Verification items for this drawing (mm, ordinates from the low corner). A direction names the side the tool comes from. Coordinates: 2 decimals unless noted, no trailing zeros. Write each loop counter-clockwise with the first axis right and the second up, starting at its lowest first coordinate (ties: lowest second). Pieces come first, ordered by that corner, then holes. Notation, with made-up numbers: (-8, 55.5) -> (48, 55.5) arc R5 cw to (48, 64.5) -> close; hole circle Ø1 at (15, -23.5). An arc over 180 degrees is marked (long way). Use CSV: the item, a comma, the result in double quotes.
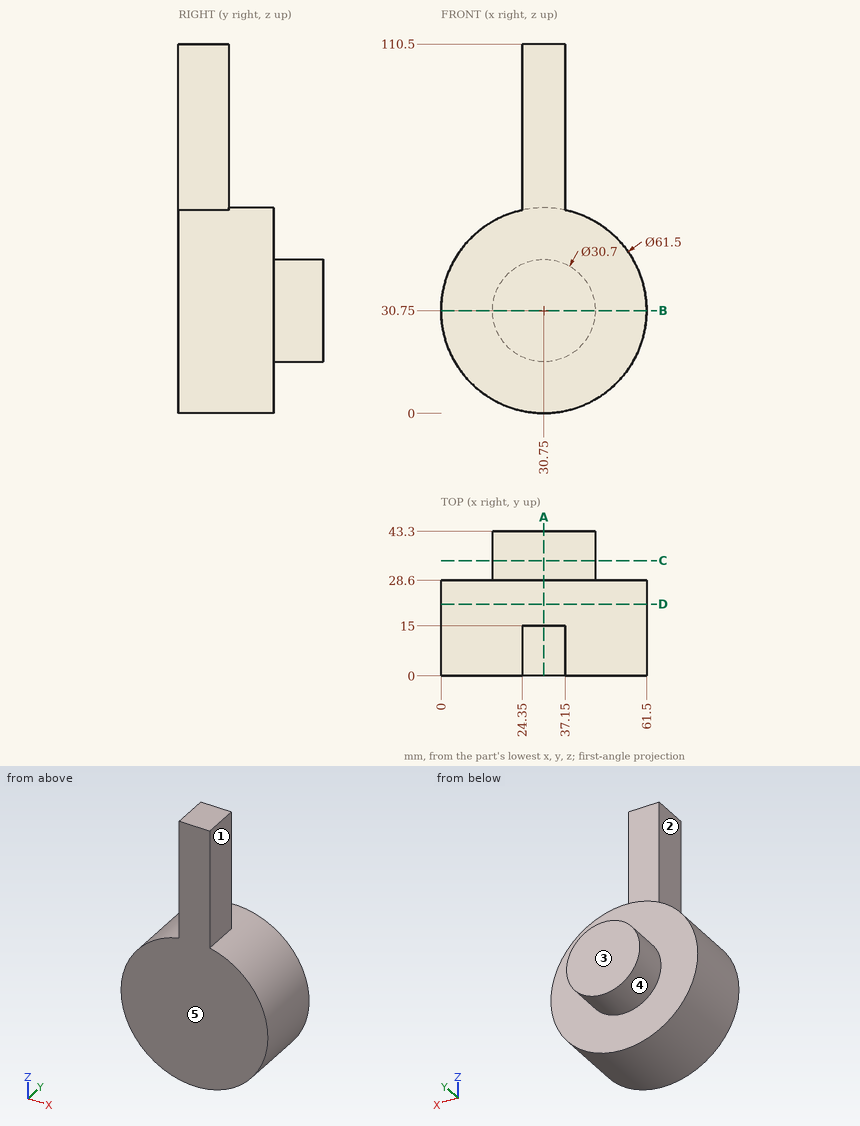
1) Cross-section at B-B (z = 30.75). Record the boundary of the cut face in (x, y), plus the area to 3 significant figures.
Return value:
outline,"(0, 0) -> (61.5, 0) -> (61.5, 28.6) -> (46.1, 28.6) -> (46.1, 43.3) -> (15.4, 43.3) -> (15.4, 28.6) -> (0, 28.6) -> close"
area,"2,210 mm2"
2) Cross-section at A-A (x = 30.75). Record the boundary of the cut face in (y, z), plus the area to 3 significant figures.
Return value:
outline,"(0, 0) -> (28.6, 0) -> (28.6, 15.4) -> (43.3, 15.4) -> (43.3, 46.1) -> (28.6, 46.1) -> (28.6, 61.5) -> (15, 61.5) -> (15, 110.5) -> (0, 110.5) -> close"
area,"2,950 mm2"
3) Gauge pin test, flat ends, axial feed: pin 1 (3 mm diameter, centred on x = 6.5, z = 34.5, fed in from +Y); pin 2 (10 mm diameter, centred on x = 29, z = 81, fed in from +Y); pin 3 (5 mm diameter, centred on y = 35, z = 32.5, fed in from -X). Record the tip position at first contact, or that the pin passes through.
Return value:
pin 1,"y = 28.6"
pin 2,"y = 15"
pin 3,"x = 15.4"
4) Scan lines: L1, parallel to X at y = 2, z = 90; L2, parallel to Z at x = 30, y = 23.5; L3, parallel to Y at x = 7, z = 49.5. Record each from-to range of solid material in increasing order.
Return value:
L1,"24.35 to 37.15"
L2,"0.01 to 61.49"
L3,"0 to 28.6"
5) Cross-section at D-D (y = 21.5). Record the boundary of the cut face in (x, z).
Return value:
outline,"circle Ø61.5 at (30.75, 30.75)"
6) Cross-section at C-C (y = 34.5). Record the boundary of the cut face in (x, z).
Return value:
outline,"circle Ø30.7 at (30.75, 30.75)"
7) Set-up check for the marked faces 1, 2, 3, 4 and 5: record each of +Z, -Z, +X, -X, +Y, -Y from which the full face is reachable in a straight line by a thin tool's end or side.
Return value:
face 1,"+Z, +X, +Y, -Y"
face 2,"+Z, -X, +Y, -Y"
face 3,"+Z, -Z, +X, -X, +Y"
face 4,"+Y"
face 5,"+Z, -Z, +X, -X, -Y"
